Design review of the part built by this model. Coordinates are the model's own, in mm. A direction names the side the tool comes from. Coordinates: 2 decimals unless noted, no trailing zeros. Write each loop counter-clockwise with the first axis right and the second up, starting at its lowest first coordinate (ties: lowest second). Pieces come first, ordered by that corner, then holes. Notation, with made-up numbers: M -28.5,75.25 L -4.5,75.25 A36 ccw -4.5,111.25 Z; hole C 14.25,78 d11. An arc over 180 degrees is marked long. Return JSON: item names as keys, results as strings. Group by question number.
```python
from build123d import *

# Parameters (mm, degrees)
SKETCH_1_W          = 96
SKETCH_1_H          = 62
EXTRUDE_1_DEPTH     = 2
SKETCH_2_W          = 55.125
SKETCH_2_H          = 18.9014
SKETCH_2_W_2        = 81
SKETCH_2_H_2        = 10.505077979
SKETCH_2_W_3        = 81.042070701
SKETCH_2_H_3        = 9.043475151
CUT_EXTRUDE_1_DEPTH = 2
SKETCH_3_W          = 48
SKETCH_3_H          = 2
CUT_EXTRUDE_2_DEPTH = 3
SKETCH_4_W          = 48
SKETCH_4_H          = 2
CUT_EXTRUDE_3_DEPTH = 3
SKETCH_5_W          = 2
SKETCH_5_H          = 31
CUT_EXTRUDE_4_DEPTH = 3
SKETCH_6_W          = 2
SKETCH_6_H          = 31
CUT_EXTRUDE_5_DEPTH = 3


with BuildPart() as part:
    # ｽｹｯﾁ1 → ﾎﾞｽ - 押し出し1 (new body)
    with BuildSketch(Plane.XY):
        with Locations((5.311186132, -2.735849057)):
            Rectangle(SKETCH_1_W, SKETCH_1_H)
    extrude(amount=EXTRUDE_1_DEPTH)

    # ｽｹｯﾁ2 → ｶｯﾄ - 押し出し1 (cut)
    with BuildSketch(Plane(origin=(0, 0, 0), x_dir=(-1, 0, 0), z_dir=(0, 0, -1))):
        with Locations((7.376313868, -20.786549057)):
            Rectangle(SKETCH_2_W, SKETCH_2_H)
        with Locations((-5.561186132, 0.116689932)):
            Rectangle(SKETCH_2_W_2, SKETCH_2_H_2)
        with Locations((-5.540150781, 18.185888519)):
            Rectangle(SKETCH_2_W_3, SKETCH_2_H_3)
    extrude(amount=-CUT_EXTRUDE_1_DEPTH, mode=Mode.SUBTRACT)

    # ｽｹｯﾁ3 → ｶｯﾄ - 押し出し2 (cut, through all)
    with BuildSketch(Plane(origin=(0, 0, 0), x_dir=(-1, 0, 0), z_dir=(0, 0, -1))):
        with Locations((-5.311186132, -32.735849057)):
            Rectangle(SKETCH_3_W, SKETCH_3_H)
    extrude(amount=-CUT_EXTRUDE_2_DEPTH, mode=Mode.SUBTRACT)

    # ｽｹｯﾁ4 → ｶｯﾄ - 押し出し3 (cut, through all)
    with BuildSketch(Plane(origin=(0, 0, 0), x_dir=(-1, 0, 0), z_dir=(0, 0, -1))):
        with Locations((-5.311186132, 27.264150943)):
            Rectangle(SKETCH_4_W, SKETCH_4_H)
    extrude(amount=-CUT_EXTRUDE_3_DEPTH, mode=Mode.SUBTRACT)

    # ｽｹｯﾁ5 → ｶｯﾄ - 押し出し4 (cut, through all)
    with BuildSketch(Plane(origin=(0, 0, 0), x_dir=(-1, 0, 0), z_dir=(0, 0, -1))):
        with Locations((41.688813868, -2.735849057)):
            Rectangle(SKETCH_5_W, SKETCH_5_H)
    extrude(amount=-CUT_EXTRUDE_4_DEPTH, mode=Mode.SUBTRACT)

    # ｽｹｯﾁ6 → ｶｯﾄ - 押し出し5 (cut, through all)
    with BuildSketch(Plane(origin=(0, 0, 0), x_dir=(-1, 0, 0), z_dir=(0, 0, -1))):
        with Locations((-52.311186132, -2.735849057)):
            Rectangle(SKETCH_6_W, SKETCH_6_H)
    extrude(amount=-CUT_EXTRUDE_5_DEPTH, mode=Mode.SUBTRACT)


solid = part.part
```
Item 1: Machinability: for faces 1 (the flat face through (-42, 12.764, 1)), 2 (the flat face through (52, -18.236, 1)), 3 (the flat face through (6, 5.369, 1)), which of the approach directions +Z, -Z, +X, -X, +Y, -Y give a long, thin tool a straight path to every point of the face, cutting with its end or side? Answer none if there is none.
Item 2: For pin 1 (2 mm diameter, centred on x = 34, y = 6, fed in from -Z), flat-tipped, find the tip position at first contact; note if it passes through.
Item 3: Add section D-D (y = 0.5). Write out the cut boundary in (x, z), plus the area to 3 significant figures.
Item 4: For line 1 (Y direction, x = -15.5, z = 0.55); line 2 (Y direction, x = 45, z = 1); line 3 (Y direction, x = -26, z = 1.25), list the stretches that pass through material, from the lowest coordinate up.
Item 5: Add section C-C (x = 43.5). Write out the cut boundary in (y, z), plus the area to 3 significant figures.
Item 6: Add section A-A (y = -25.5). Write out the cut boundary in (x, z).
Item 7: Add section B-B (z = 0.6). Count the separate pieces of the cut face and the enclosed holes in it, plus the area to 3 significant figures.
Item 8: The part is to be moulded in two halves that separate along X. For faces 4 (the flat face through (6, 13.664, 1)), 5 (the flat face through (-7, -30.237, 1)), 6 (the flat face through (-42.689, 20, 1)), 7 (the flat face through (5, -9, 0)), say which applies: pulls with the +X half, pulls with the -X half, needs draft (parallel to the pull), parting line crosses it, or undercut.
Geometry check:
{
 "1": {"face 1": "+Z, -Z, -X", "face 2": "+Z, -Z, +X", "face 3": "+Z, -Z"},
 "2": {"pin 1": "z = 0"},
 "3": {"outline": "M -40.69,0 L -34.94,0 L -34.94,2 L -40.69,2 Z; M 46.06,0 L 51.31,0 L 51.31,2 L 46.06,2 Z", "area": "22.0 mm^2"},
 "4": {"line 1": "-31.74 to -30.24, -11.34 to -5.14, 5.37 to 13.66, 22.71 to 26.26", "line 2": "-33.74 to -5.14, 5.37 to 13.66, 22.71 to 28.26", "line 3": "-33.74 to -30.24, -11.34 to -5.14, 5.37 to 13.66, 22.71 to 28.26"},
 "5": {"outline": "M -33.74,0 L -5.14,0 L -5.14,2 L -33.74,2 Z; M 5.37,0 L 13.66,0 L 13.66,2 L 5.37,2 Z; M 22.71,0 L 28.26,0 L 28.26,2 L 22.71,2 Z", "area": "84.9 mm^2"},
 "6": {"outline": "M -42.69,0 L -34.94,0 L -34.94,2 L -42.69,2 Z; M 20.19,0 L 53.31,0 L 53.31,2 L 20.19,2 Z"},
 "7": {"separate pieces": "1", "enclosed holes": "3", "area": "3,010 mm^2"},
 "8": {"face 4": "undercut", "face 5": "undercut", "face 6": "pulls with the -X half", "face 7": "needs draft"}
}
